Source: three-view drawing plus pictorial views. Frame: mm from the lowest corner of the part. A direction names the side the tool comes from. Coordinates: 2 decimals unless noted, no trailing zeros. Order: outer loops, then holes, each group sorted by start corner. A loop starts at its lowest first (then second) coordinate and runs counter-clockwise, first axis right, second up. Notation, with made-up numbers: M 80.25,8 L 94.25,8 A24 ccw 94.25,25 Z; hole C 4,62.5 d7. An arc over 180 degrees is marked long. Use CSV: the item, a comma, the result in double quotes. Start each with the question number.
Q1. Section query B-B, the plane y = 12.75. Output: boundary loops of the cut face in (x, z), and give its area (3 significant figures).
Q2. Section query D-D, the plane y = 3.75. Output: boundary loops of the cut face in (x, z), and give its area (3 significant figures).
Q3. Access query for the marked faces 3 and 4. Directions: +Z, -Z, +X, -X, +Y, -Y. A direction counts if a zero-diameter tool reaches every point of the face in a straight line with its end or side. Return the directions, or none.
Q4. Ray query, probe 1 along Y at (x, z) = (14, 6.8); probe 2 along Z at (x, y) = (7.75, 22.25); probe 3 along X at (y, z) = (8.25, 4). Return the intervals inside material, ascending.
Q5. Mould query, pull axis Y, two halves, no side actions, for the marked faces 1 and 2. Classes: +Y half, -Y half, draft (parallel to the pull), parting line (faces both ways), or undercut.
Q6. First-contact query: P1, Ø1.5, axis at y = 24.5, z = 4, coming from the -X side; P2, Ø5, axis at x = 22, y = 19, coming from the +Z side; P3, Ø3, axis at x = 19.5, z = 5.5, coming from the +Y side; P4, Ø4, axis at y = 23.5, z = 2, coming from the -X side. Flat tips, straight axial feed; report the tip coordinate or a pass-through.
Q7. Section query C-C, the plane z = 4.5. Output: boundary loops of the cut face in (x, y), and give its area (3 significant figures).
Q8. Section query A-A, the plane x = 14. Output: boundary loops of the cut face in (y, z), and give its area (3 significant figures).
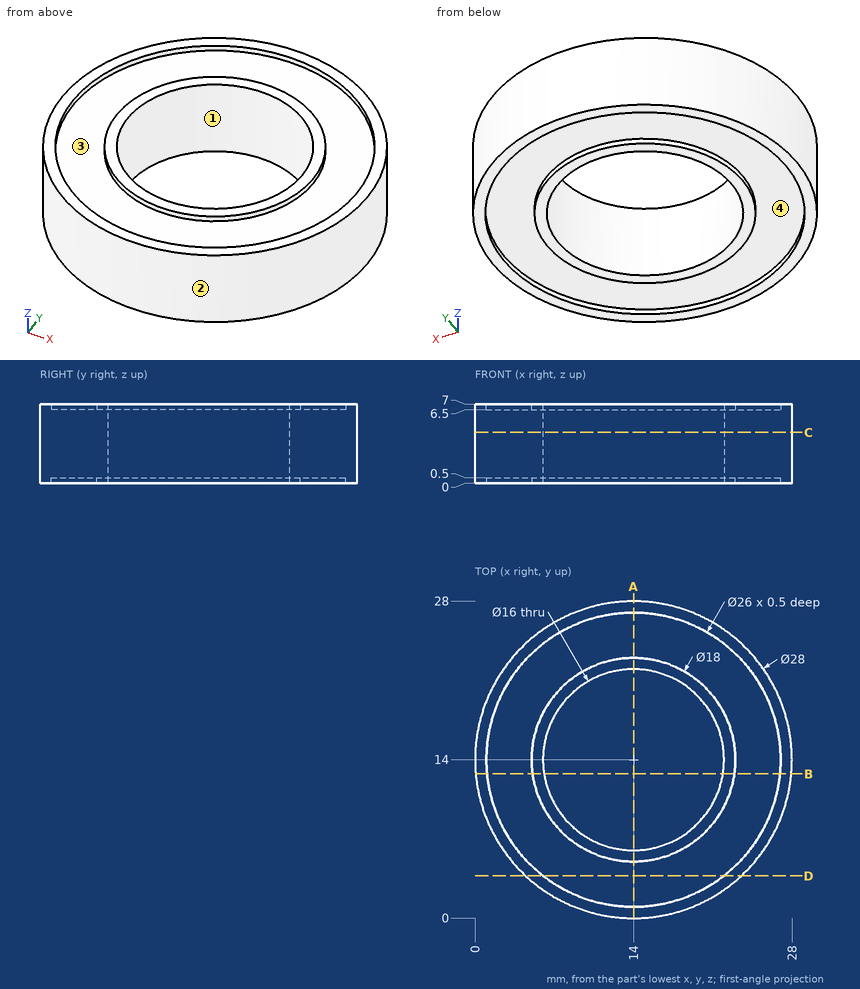
Responses:
1,outline,"M 0.06,0 L 1.06,0 L 1.06,0.5 L 5.09,0.5 L 5.09,0 L 6.1,0 L 6.1,7 L 5.09,7 L 5.09,6.5 L 1.06,6.5 L 1.06,7 L 0.06,7 Z; M 21.9,0 L 22.91,0 L 22.91,0.5 L 26.94,0.5 L 26.94,0 L 27.94,0 L 27.94,7 L 26.94,7 L 26.94,6.5 L 22.91,6.5 L 22.91,7 L 21.9,7 Z"
1,area,"76.5 mm²"
2,outline,"M 4.46,0 L 6,0 L 6,0.5 L 22,0.5 L 22,0 L 23.54,0 L 23.54,7 L 22,7 L 22,6.5 L 6,6.5 L 6,7 L 4.46,7 Z"
2,area,"118 mm²"
3,face 3,"+Z"
3,face 4,"-Z"
4,probe 1,"y = 0 to 1, 5 to 6, 22 to 23, 27 to 28"
4,probe 2,"z = 0.5 to 6.5"
4,probe 3,"x = 1.24 to 8.44, 19.56 to 26.76"
5,face 1,"undercut"
5,face 2,"parting line"
6,P1,"stops at x = 3.95"
6,P2,"stops at z = 7"
6,P3,"stops at y = 27.42"
6,P4,"stops at x = 2.18"
7,outline,"C 14,14 d28; hole C 14,14 d16"
7,area,"415 mm²"
8,outline,"M 0,0 L 1,0 L 1,0.5 L 5,0.5 L 5,0 L 6,0 L 6,7 L 5,7 L 5,6.5 L 1,6.5 L 1,7 L 0,7 Z; M 22,0 L 23,0 L 23,0.5 L 27,0.5 L 27,0 L 28,0 L 28,7 L 27,7 L 27,6.5 L 23,6.5 L 23,7 L 22,7 Z"
8,area,"76.0 mm²"
